```python
from build123d import *

# Parameters (mm, degrees)
IZIM1_R                     = 75
IZIM1_R_2                   = 100
Y_KSEKLIK_EKSTR_ZYON3_DEPTH = 250
KES_EKSTR_ZYON2_DEPTH       = 240
IZIM4_R                     = 18
KES_EKSTR_ZYON3_DEPTH       = 240
DAIRESEL_KAPLAMA1_COUNT     = 4


with BuildPart() as part:
    # Çizim1 → Yükseklik-Ekstrüzyon3 (new body)
    with BuildSketch(Plane(origin=(0, 0, 0), x_dir=(1, 0, 0), z_dir=(0, 1, 0))):
        with BuildLine():
            Line((326.203305187, 550), (-325, 550))
            ThreePointArc((-325, 550), (-709.099025767, 709.099025767), (-550, 325))
            Line((-550, 325), (-550, -324.872993427))
            ThreePointArc((-550, -324.872993427), (-709.188832976, -709.188832976), (-324.872993427, -550))
            Line((-324.872993427, -550), (326.203305187, -550))
            ThreePointArc((326.203305187, -550), (708.248160509, -708.248160509), (550, -326.203305187))
            Line((550, -326.203305187), (550, 326.203305187))
            ThreePointArc((550, 326.203305187), (708.248160509, 708.248160509), (326.203305187, 550))
        make_face()
        with Locations(Location((0, 0, 0), (0, 0, 270))):
            Circle(IZIM1_R, mode=Mode.SUBTRACT)
        with Locations(Location((-550, 550, 0), (0, 0, 270))):
            Circle(IZIM1_R_2, mode=Mode.SUBTRACT)
        with Locations(Location((-550, -550, 0), (0, 0, 270))):
            Circle(IZIM1_R_2, mode=Mode.SUBTRACT)
        with Locations(Location((550, 550, 0), (0, 0, 270))):
            Circle(IZIM1_R_2, mode=Mode.SUBTRACT)
        with Locations(Location((550, -550, 0), (0, 0, 270))):
            Circle(IZIM1_R_2, mode=Mode.SUBTRACT)
    extrude(amount=Y_KSEKLIK_EKSTR_ZYON3_DEPTH)

    # Çizim2 → Kes-Ekstrüzyon2 (cut)
    with BuildSketch(Plane(origin=(0, 250, 0), x_dir=(1, 0, 0), z_dir=(0, 1, 0))):
        with BuildLine():
            Line((-550, 325), (-550, -324.872993427))
            ThreePointArc((-550, -324.872993427), (-415.406896151, 0.063503286), (-550, 325))
        make_face()
        with BuildLine():
            Line((-324.872993427, -550), (326.203305187, -550))
            ThreePointArc((326.203305187, -550), (0.66515588, -415.157683487), (-324.872993427, -550))
        make_face()
        with BuildLine():
            Line((-325, 550), (326.203305187, 550))
            ThreePointArc((326.203305187, 550), (0.601652594, 415.131379565), (-325, 550))
        make_face()
        with BuildLine():
            Line((550, 326.203305187), (550, -326.203305187))
            ThreePointArc((550, -326.203305187), (414.882166901, 0), (550, 326.203305187))
        make_face()
    extrude(amount=-KES_EKSTR_ZYON2_DEPTH, mode=Mode.SUBTRACT)

    # Çizim4 → Kes-Ekstrüzyon3 (cut)
    with BuildSketch(Plane(origin=(0, 10, 0), x_dir=(1, 0, 0), z_dir=(0, 1, 0))):
        with Locations(Location((-494.284737224, 0.063503286, 0), (0, 0, 270))):
            Circle(IZIM4_R)
    kes_ekstr_zyon3 = extrude(amount=-KES_EKSTR_ZYON3_DEPTH, mode=Mode.SUBTRACT)

    # Dairesel Kaplama1: Kes-Ekstrüzyon3 ×4 about axis
    dairesel_kaplama1_axis = Axis((0, 0, 0), (0, 1, 0))
    for i in range(1, DAIRESEL_KAPLAMA1_COUNT):
        add(kes_ekstr_zyon3.rotate(dairesel_kaplama1_axis, i * 360 / DAIRESEL_KAPLAMA1_COUNT), mode=Mode.SUBTRACT)


solid = part.part
```
Source: CAD feature listing. Evaluate the final solid. Frame: model axes, mm. A direction names the side the tool comes from. Give positions to 0.01 mm unless a question says otherwise; leave off trailing zeros. Loops run counter-clockwise (first coordinate to the right, second up) from the corner with the lowest first, then second, coordinate; pieces in that order, holes last. Notation, with made-up numbers: (21.25, -25) -> (28.25, -25) arc R17 ccw to (28.25, 2) -> close; hole circle Ø9 at (73.25, 28). An arc over 180 degrees is marked (long way). Use a Markdown table: item, result. Add a question column.
(1) Ray query, line 1 (X direction, y = 141, z = 550); line 2 (X direction, y = 192, z = 0); line 3 (Z direction, x = -631, y = 139.5). Return the intervals inside material, ascending.
(2) Section query B-B (z = 0). Output: boundary loops of the cut face in (x, y), then the cut area to 3 significant figures.
(3) First-contact query: pin 1 Ø11 at (y, z) = (6.5, -43) entering from +X; pin 2 Ø5 at (x, y) = (-386, 178.5) entering from -Z; pin 3 Ø11 at (y, z) = (7, 110.5) entering from -X; pin 4 Ø10 at (x, z) = (548.5, -289) entering from -Y. Flat tips, straight axial feed; report the tip coordinate or a pass-through.
(4) Section query C-C (y = 230.5). Output: boundary loops of the cut face in (x, z), then the cut area to 3 significant figures.
(5) Section query A-A (x = 0). Output: boundary loops of the cut face in (y, z).
(6) Pull-direction query (Z, two-part tool) for faces 1 (the face through (5.66, 131.68, -415.16)), 2 (the face through (-184, 250, -11)), 3 (the face through (-45.636, 123.25, -59.517)); classes: +Z half, -Z half, draft (parallel to the pull), parting line (faces both ways), or undercut.
(7) Section query D-D (x = -615.5). Output: boundary loops of the cut face in (y, z), then the cut area to 3 significant figures.
(8) Access query for faces 4 (the face through (414.91, 131.68, 5.07)), 5 (the face through (-514, 10, -5)), 6 (the face through (713.381, 123.25, -702.943)), 7 (the face through (-4, 10, 467)), 8 (the face through (5, 10, -513)). Directions: +Z, -Z, +X, -X, +Y, -Y. A direction counts if a zero-diameter tool reaches every point of the face in a straight line with its end or side. Return the directions, or none.
Checked values:
| question | item | result |
|---|---|---|
| 1 | line 1 | -775.13 to -650, -450 to -324.87, 326.2 to 450, 650 to 773.8 |
| 1 | line 2 | -415.41 to -75, 75 to 414.88 |
| 1 | line 3 | -759.91 to -608.64, -491.36 to -340.09, 339.95 to 491.36, 608.64 to 760.05 |
| 2 | outline | (-550, 0) -> (-512.28, 0) -> (-512.28, 10) -> (-550, 10) -> close; (-476.28, 0) -> (-75, 0) -> (-75, 250) -> (-415.41, 250) -> (-415.41, 10) -> (-476.28, 10) -> close; (75, 0) -> (476.28, 0) -> (476.28, 10) -> (414.88, 10) -> (414.88, 250) -> (75, 250) -> close; (512.28, 0) -> (550, 0) -> (550, 10) -> (512.28, 10) -> close |
| 2 | area | 172,000 mm^2 |
| 3 | pin 1 | x = 550 |
| 3 | pin 2 | z = -706.66 |
| 3 | pin 3 | x = -550 |
| 3 | pin 4 | y = 0 |
| 4 | outline | (-550, -325) arc R225 ccw (long way) to (-325, -550) arc R460.47 cw to (326.2, -550) arc R223.8 ccw (long way) to (550, -326.2) arc R461.32 cw to (550, 326.2) arc R223.8 ccw (long way) to (326.2, 550) arc R460.38 cw to (-324.87, 550) arc R225.13 ccw (long way) to (-550, 324.87) arc R459.53 cw to start; hole circle Ø200 at (-550, -550); hole circle Ø200 at (-550, 550); hole circle Ø150 at (0, 0); hole circle Ø200 at (550, -550); hole circle Ø200 at (550, 550) |
| 4 | area | 1,300,000 mm^2 |
| 5 | outline | (0, -550) -> (10, -550) -> (10, -512.28) -> (0, -512.28) -> close; (0, -476.28) -> (10, -476.28) -> (10, -415.13) -> (250, -415.13) -> (250, -75) -> (0, -75) -> close; (0, 75) -> (250, 75) -> (250, 415.16) -> (10, 415.16) -> (10, 476.28) -> (0, 476.28) -> close; (0, 512.28) -> (10, 512.28) -> (10, 550) -> (0, 550) -> close |
| 6 | face 1 | -Z half |
| 6 | face 2 | draft |
| 6 | face 3 | undercut |
| 7 | outline | (0, -765.26) -> (250, -765.26) -> (250, -625.56) -> (0, -625.56) -> close; (0, -474.44) -> (250, -474.44) -> (250, -334.74) -> (0, -334.74) -> close; (0, 334.61) -> (250, 334.61) -> (250, 474.44) -> (0, 474.44) -> close; (0, 625.56) -> (250, 625.56) -> (250, 765.39) -> (0, 765.39) -> close |
| 7 | area | 140,000 mm^2 |
| 8 | face 4 | +X, +Y |
| 8 | face 5 | -X, +Y |
| 8 | face 6 | +Y, -Y |
| 8 | face 7 | +Z, +Y |
| 8 | face 8 | -Z, +Y |
